Input: part model. Units: mm. Frame: model coordinates. Give positions to 0.01 mm unless a question says otherwise; leave off trailing zeros. Order: outer loops, then holes, each group sorted by start corner. A loop starts at its lowest first (then second) coordinate and runs counter-clockwise, first axis right, second up. Notation, with made-up numbers: M 43.25,17 L 50.25,17 A22 ccw 50.25,23 Z; hole C 24,41.25 d10. An arc over 180 degrees is marked long. Use a Markdown table: item, result.
from build123d import *

# Parameters (mm, degrees)
F0_W     = 152.4
F0_H     = 1447.8
F1_DEPTH = 254
F3_DEPTH = 25.4
F4_R     = 6.35
F5_DEPTH = 12.7


with BuildPart() as f1:
    # F0 (on Top) → F1 (new body)
    with BuildSketch(Plane.XY):
        with Locations((37.643603, 672.619554)):
            Rectangle(F0_W, F0_H)
    extrude(amount=F1_DEPTH)

    # F2 (on face) → F3 (join)
    with BuildSketch(Plane.XY.offset(254)):
        with BuildLine():
            ThreePointArc((37.643603, 475.769554), (42.133731, 477.629426), (43.993603, 482.119554))
            ThreePointArc((43.993603, 482.119554), (42.133731, 486.609682), (37.643603, 488.469554))
            Line((37.643603, 488.469554), (37.643603, 475.769554))
        make_face()
        with BuildLine():
            ThreePointArc((51.931103, 863.119554), (27.540815, 873.222342), (37.643603, 848.832054))
            ThreePointArc((37.643603, 848.832054), (47.746391, 853.016766), (51.931103, 863.119554))
        make_face()
        with BuildLine():
            Line((37.643603, 475.769554), (37.643603, 488.469554))
            ThreePointArc((37.643603, 488.469554), (31.293603, 482.119554), (37.643603, 475.769554))
        make_face()
    extrude(amount=F3_DEPTH)

    # F4 (on face) → F5 (join)
    with BuildSketch(Plane.XZ.offset(51.280446)):
        with Locations((37.643603, 6.35)):
            Circle(F4_R)
        with BuildLine():
            ThreePointArc((5.893603, 247.65), (12.243603, 241.3), (18.593603, 247.65))
            ThreePointArc((18.593603, 247.65), (12.243603, 254), (5.893603, 247.65))
        make_face()
    extrude(amount=F5_DEPTH)


solid = f1.part
1) First-contact query: pin 1 Ø5 at (x, z) = (14, 172.5) entering from -Y; pin 2 Ø4 at (x, y) = (86, 899) entering from +Z. Flat tips, straight axial feed; report the tip coordinate or a pass-through.
Response values:
| item | result |
|---|---|
| pin 1 | stops at y = -51.28 |
| pin 2 | stops at z = 254 |
2) Material intervals for line 1 (Y direction, x = -4, z = 70.5); line 2 (Z direction, x = 72.5, y = 1126.5), sorted ascending. Write a range as from..to.
Response values:
| item | result |
|---|---|
| line 1 | y = -51.28..1396.52 |
| line 2 | z = 0..254 |
3) Cut plane B-B on x = 89.5. Return loops of the section in (y, z).
Response values:
| item | result |
|---|---|
| outline | M -51.28,0 L 1396.52,0 L 1396.52,254 L -51.28,254 Z |
4) Cut plane A-A on y = 829.5. Return loops of the section in (x, z), and give its area (3 significant figures).
Response values:
| item | result |
|---|---|
| outline | M -38.56,0 L 113.84,0 L 113.84,254 L -38.56,254 Z |
| area | 38,700 mm² |
